Can you work these out from the model? Positions are in its coordinate system, mm. Face numbers are marked on the shaded views. A direction names the side the tool comes from. Round coordinates to 2 decimals unless told otherwise and drop trailing zeros. Loops run counter-clockwise (first coordinate to the right, second up) from the corner with the lowest first, then second, coordinate; pieces in that order, holes last. Notation, with made-up numbers: (-0.75, 85) -> (9.25, 85) arc R25 cw to (9.25, 110) -> close; hole circle Ø7 at (11.25, -36). An arc over 180 degrees is marked (long way). Write item = value, one per line.
from build123d import *

# Parameters (mm, degrees)
PAD011_DEPTH    = 10.5
POCKET010_DEPTH = 5
FILLET005_R     = 1


with BuildPart() as part:
    # Sketch055 → Pad011 (new body, symmetric)
    with BuildSketch(Plane.YZ):
        Polygon((23.8941280101, -22.635866082), (28.6951768598, -25.3191346005), (27.2315758497, -27.9378885186), (22.430527, -25.25462), align=None)
    extrude(amount=PAD011_DEPTH, both=True)

    # Sketch056 (on Face1 of Pad011) → Pocket010 (cut)
    with BuildSketch(Plane(origin=(0, -3.9527461257, -7.0724666982), x_dir=(0, -0.8729179727, 0.4878670034), z_dir=(0, 0.4878670034, 0.8729179727))):
        with BuildLine():
            Line((-36.7009059356, 10), (-32.6009059356, 10))
            ThreePointArc((-32.4009059356, 9.8), (-32.4594845794, 9.9414213562), (-32.6009059356, 10))
            Line((-32.4009059356, 9.8), (-32.4009059356, -9.8))
            ThreePointArc((-32.6009059356, -10), (-32.4594845794, -9.9414213562), (-32.4009059356, -9.8))
            Line((-32.6009059356, -10), (-36.7009059356, -10))
            ThreePointArc((-36.9009059356, -9.8), (-36.8423272919, -9.9414213562), (-36.7009059356, -10))
            Line((-36.9009059356, -9.8), (-36.9009059356, 9.8))
            ThreePointArc((-36.7009059356, 10), (-36.8423272919, 9.9414213562), (-36.9009059356, 9.8))
        make_face()
    extrude(amount=-POCKET010_DEPTH, mode=Mode.SUBTRACT)

    # Fillet005
    fillet005_edges = [part.edges().sort_by_distance(p)[0] for p in [
        (10.5, 27.963376, -26.628512),
        (10.5, 23.162328, -23.945243),
        (-10.5, 27.963376, -26.628512),
        (-10.5, 23.162328, -23.945243),
    ]]
    fillet(fillet005_edges, radius=FILLET005_R)


solid = part.part
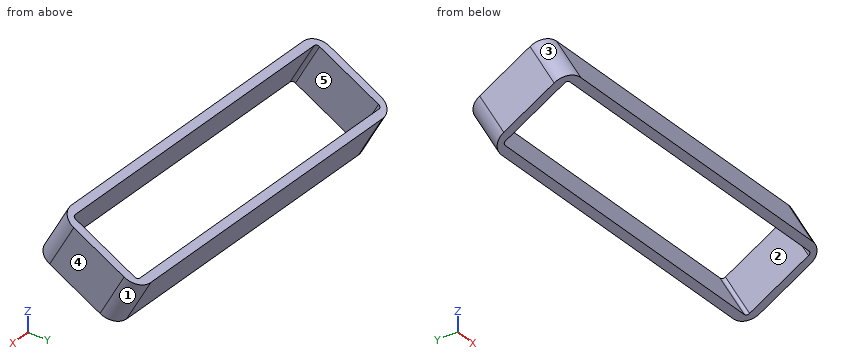
1. We'd pull the mould along X, two halves only. Please class the marked faces 1, 2 and 3: released by +X, released by -X, zero draft, split by the parting line, or undercut.
Entries:
face_1 = released by +X
face_2 = undercut
face_3 = released by -X
2. For the marked faces 4 and 5, which set-ups out of +Z, -Z, +X, -X, +Y, -Y let a thin tool reach every point of the face, with its end or its side?
Entries:
face_4 = +Z, -Z, +X, +Y, -Y
face_5 = none
3. Suppose I cut it at A-A, the plane x = -2. List the corners of the cut face in (y, z) for me.
Entries:
outline = (22.43, -25.25) -> (22.87, -25.5) -> (24.33, -22.88) -> (23.89, -22.64) -> close; (26.8, -27.69) -> (27.23, -27.94) -> (28.7, -25.32) -> (28.26, -25.08) -> close
4. Suppose I cut it at B-B, the plane y = 26. List the corners of the cut face in (x, z) for me, and give its area (3 significant figures).
Entries:
outline = (-10.5, -27.25) -> (-10, -27.25) -> (-10, -23.81) -> (-10.5, -23.81) -> close; (10, -27.25) -> (10.5, -27.25) -> (10.5, -23.81) -> (10, -23.81) -> close
area = 3.44 mm²
5. I need wall thicknesses on line 1 (X direction, y = 26.5, z = -24.65); line 2 (Y direction, x = -5.5, z = -24.5); line 3 (Y direction, x = 1, z = -23). Which ranges of each line are inside material? Lowest first, please. Write a range as [from, to].
Entries:
line_1 = [-10.5, -10], [10, 10.5]
line_2 = [22.85, 23.43]
line_3 = [23.69, 24.26]
6. I'm going to push flat-ended pins straight in: pin 1 (1 mm diameter, centred on x = 5.5, z = -23.5, fed in from +Y); pin 2 (1 mm diameter, centred on x = -2, y = 24, fed in from +Z). Where does each tip first touch, or does it pass through?
Entries:
pin_1 = 24.26
pin_2 = -22.64
